Autodesk Inventor part; units mm, degrees
ref_plane "YZ Plane" through (0, 0, 0) normal (1, 0, 0) x (0, 1, 0)
ref_plane "XZ Plane" through (0, 0, 0) normal (0, 1, 0) x (-1, 0, 0)
ref_plane "XY Plane" through (0, 0, 0) normal (0, 0, 1) x (1, 0, 0)
sketch "Sketch1" plane through (0, 0, 0) normal (0, 1, 0) x (-1, 0, 0)
  circle A0 centre (0, 0) radius 19.05
  dimension "d0" = 38.1
extrude "Extrusion1" add sketch "Sketch1" along normal blind 3.175
sketch "Sketch2" plane through (0, 3.175, 0) normal (0, 1, 0) x (1, 0, 0)
  circle A0 centre (0, 0) radius 6.1595
  dimension "d3" = 12.319
extrude "Extrusion2" add sketch "Sketch2" along normal blind 9.525
fillet "Fillet1" radius 1.5875 1 edges at (-6.1595, 3.175, 0)
fillet "Fillet2" radius 3.175 1 edges at (-6.1595, 12.7, 0)
fillet "Fillet3" radius 1.5875 1 edges at (19.05, 3.175, 0)
properties part number "Feet Cap"
CAD build for the part. Positions are in the model's coordinates, mm. A direction names the side the tool comes from. Round coordinates to 2 decimals unless told otherwise and drop trailing zeros. Write each loop counter-clockwise with the first axis right and the second up, starting at its lowest first coordinate (ties: lowest second). Pieces come first, ordered by that corner, then holes.
Item 1: Band-saw the part on A-A on y = 6.25. Write the cut outline in (x, z).
Filled in:
outline: circle Ø12.32 at (0, 0)
Item 2: Drop flat-ended pins along their axis: pin 1 Ø5 at (y, z) = (6, 5) entering from -X; pin 2 Ø1 at (x, z) = (11.5, -9) entering from +Y (3 decimals); pin 3 Ø5 at (x, y) = (9, 11) entering from -Z. Give the stop position or say it passes through.
Filled in:
pin 1: stops at x = -5.63
pin 2: stops at y = 3.175
pin 3: passes through
Item 3: Drill centre lines: L1, parallel to Y at x = -11.5, z = -10 (3 decimals); L2, parallel to Z at x = -13.5, y = 0.75; L3, parallel to Z at x = -9, y = 1.25. Where is each one in solid material? Low to high.
Filled in:
L1: y = 0 to 3.175
L2: z = -13.44 to 13.44
L3: z = -16.79 to 16.79
Item 4: Tool access for faces 1 (the flat face through (-4, 3.175, -8)), 2 (the flat face through (0, 12.7, 0)): list every direction of +Z, -Z, +X, -X, +Y, -Y with a clear straight run to the whole face (end or side of a thin tool).
Filled in:
face 1: +Y
face 2: +Z, -Z, +X, -X, +Y
